For this review, take the finished solid that the model builds, in its own axes (mm). A direction names the side the tool comes from. Coordinates: 2 decimals unless noted, no trailing zeros. Write each loop counter-clockwise with the first axis right and the second up, starting at its lowest first coordinate (ties: lowest second). Pieces come first, ordered by that corner, then holes. Notation, with made-up numbers: M 75.25,-3 L 90.25,-3 A20 ccw 90.25,35 Z; hole C 40.5,60 d10. An arc over 180 degrees is marked long. Return JSON: item names as keys, results as strings.
```python
from build123d import *

# Parameters (mm, degrees)
SKETCH12_W                         = 25.4
SKETCH12_H                         = 50.8
SKETCH12_W_2                       = 20.32
SKETCH12_H_2                       = 45.72
RECTANGULAR_TUBE_2IN_X_1IN_1_DEPTH = 50.8
F_1_1_8_CLEARANCE_HOLE1_D          = 28.97124


with BuildPart() as part:
    # Sketch12 → Rectangular tube 2IN X 1IN(1) (new body)
    with BuildSketch(Plane(origin=(-25.4, 0, -12.7), x_dir=(0, 0, 1), z_dir=(0, 1, 0))):
        with Locations((12.7, 25.4)):
            Rectangle(SKETCH12_W, SKETCH12_H)
        with Locations((12.7, 25.4)):
            Rectangle(SKETCH12_W_2, SKETCH12_H_2, mode=Mode.SUBTRACT)
    extrude(amount=RECTANGULAR_TUBE_2IN_X_1IN_1_DEPTH)

    # 1-1/8 Clearance Hole1 (through all)
    with Locations(Plane.XY.offset(12.7)):
        with Locations((0, 25.4)):
            Hole(F_1_1_8_CLEARANCE_HOLE1_D / 2)


solid = part.part
```
1. We need section D-D (y = 9). State the section outline as (x, z) points, plus the area to 3 significant figures.
Checks:
{"outline": "M -25.4,-12.7 L 25.4,-12.7 L 25.4,12.7 L -25.4,12.7 Z; hole M -22.86,-10.16 L 22.86,-10.16 L 22.86,10.16 L -22.86,10.16 Z", "area": "361 mm2"}
2. Clearance check with a flat-ended pin moving along its axis: pin 1 Ø10 at (x, y) = (1, 30) entering from +Z. State where the tip first meets the part, or that it passes through.
Checks:
{"pin 1": "through"}
3. We need section B-B (x = 0). State the section outline as (y, z) points.
Checks:
{"outline": "M 0,-12.7 L 10.91,-12.7 L 10.91,-10.16 L 0,-10.16 Z; M 0,10.16 L 10.91,10.16 L 10.91,12.7 L 0,12.7 Z; M 39.89,-12.7 L 50.8,-12.7 L 50.8,-10.16 L 39.89,-10.16 Z; M 39.89,10.16 L 50.8,10.16 L 50.8,12.7 L 39.89,12.7 Z"}
4. For faces 1 (the face through (2, 0, -10.4)), 2 (the face through (10, 14, 10.16)), list the 3-axis set-ups (+Z, -Z, +X, -X, +Y, -Y) from which the entire face can be reached by the end or side of a thin tool; tool diameter is ignored.
Checks:
{"face 1": "+Z, -Z, +X, -X, -Y", "face 2": "+Y, -Y"}
5. Draft analysis for pull direction X (two halves, no side actions). For faces 3 (the face through (11, 14, 12.7)), 4 (the face through (-25.4, 25, 0)), 5 (the face through (10, 14, -10.16)), state which applies: +X half, -X half, draft (parallel to the pull), parting line (faces both ways), or undercut.
Checks:
{"face 3": "draft", "face 4": "-X half", "face 5": "undercut"}
6. We need section C-C (y = 25.4). State the section outline as (x, z) points.
Checks:
{"outline": "M -25.4,-12.7 L -14.49,-12.7 L -14.49,-10.16 L -22.86,-10.16 L -22.86,10.16 L -14.49,10.16 L -14.49,12.7 L -25.4,12.7 Z; M 14.49,-12.7 L 25.4,-12.7 L 25.4,12.7 L 14.49,12.7 L 14.49,10.16 L 22.86,10.16 L 22.86,-10.16 L 14.49,-10.16 Z"}
7. Wall thickness on L1, parallel to X at y = 26, z = 7; L2, parallel to Y at x = 0, z = 10.8; L3, parallel to Z at x = -18, y = 18: over which ranges is each line inside the solid? List them lowest first. Write a range as from..to.
Checks:
{"L1": "-25.4..-22.86, 22.86..25.4", "L2": "0..10.91, 39.89..50.8", "L3": "-12.7..-10.16, 10.16..12.7"}
8. We need section A-A (z = -4.5). State the section outline as (x, y) points.
Checks:
{"outline": "M -25.4,0 L -22.86,0 L -22.86,50.8 L -25.4,50.8 Z; M 22.86,0 L 25.4,0 L 25.4,50.8 L 22.86,50.8 Z"}
